Answer from the drawing. Dimensions are ordinates in mm from the lowest x, y and z of the part. Round coordinates to 2 decimals unless told otherwise and drop trailing zeros. Order: outer loops, then holes, each group sorted by start corner. A loop starts at its lowest first (then second) coordinate and runs counter-clockwise, first axis right, second up. Notation, with made-up numbers: (-17.75, -29) -> (5.25, -29) arc R10 cw to (5.25, -18) -> close; hole circle Ø3 at (9, -9). An arc over 180 degrees is marked (long way). Use a Markdown table: item, result. Add a question column.
Item 1: A cutting plane is placed at C-C, the plane y = 100. Determine the outline of the cut face in (x, z).
Item 2: A cutting plane is placed at A-A, the plane y = 40. Determine the outline of the cut face in (x, z).
Item 3: A cutting plane is placed at B-B, the plane x = 48. Determine the outline of the cut face in (y, z).
Item 4: Flat-ended cylindrical pins translate along their axes: P1, Ø5, axis at x = 38.94, y = 66.19, coming from the +Z side; P2, Ø1.6, axis at x = 82, z = 4, coming from the -Y side; P3, Ø3.5, axis at x = 13, z = 4, coming from the +Y side. Find the tip coordinate at first contact, or state that the pin passes through.
Item 5: A cutting plane is placed at D-D, the plane z = 5.5. Give the number of separate pieces and of enclosed holes in the cut face, plus the area to 3 significant figures.
Item 6: Find the intervals of material crossed by L1, parallel to Z at x = 83, y = 16; L2, parallel to Y at x = 48, z = 6.75; L3, parallel to X at y = 76, z = 6.75 (1 decimal), in increasing order. Write a range as [from, to].
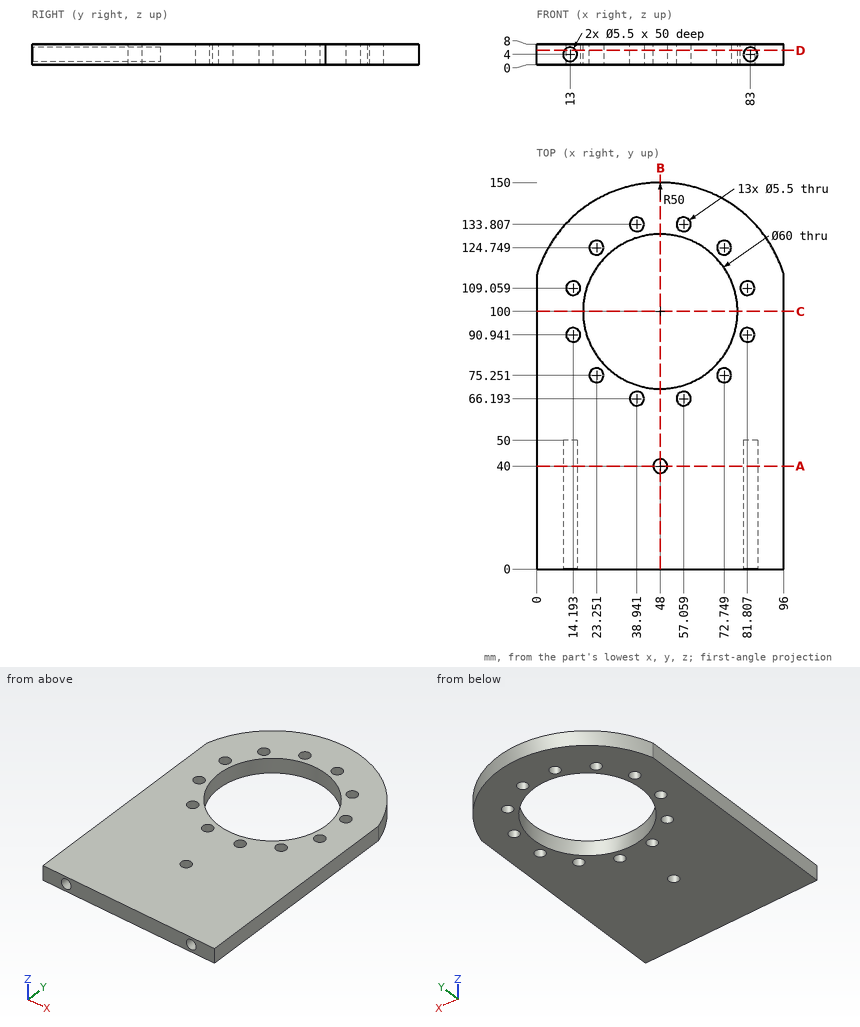
Reported:
| question | item | result |
|---|---|---|
| 1 | outline | (0, 0) -> (18, 0) -> (18, 8) -> (0, 8) -> close; (78, 0) -> (96, 0) -> (96, 8) -> (78, 8) -> close |
| 2 | outline | (0, 0) -> (45.25, 0) -> (45.25, 8) -> (0, 8) -> close; (50.75, 0) -> (96, 0) -> (96, 8) -> (50.75, 8) -> close; hole circle Ø5.5 at (13, 4); hole circle Ø5.5 at (83, 4) |
| 3 | outline | (0, 0) -> (37.25, 0) -> (37.25, 8) -> (0, 8) -> close; (42.75, 0) -> (70, 0) -> (70, 8) -> (42.75, 8) -> close; (130, 0) -> (150, 0) -> (150, 8) -> (130, 8) -> close |
| 4 | P1 | through |
| 4 | P2 | y = 50 |
| 4 | P3 | y = 137.34 |
| 5 | separate pieces | 1 |
| 5 | enclosed holes | 14 |
| 5 | area | 9,890 mm² |
| 6 | L1 | [0, 1.25], [6.75, 8] |
| 6 | L2 | [0, 37.25], [42.75, 70], [130, 150] |
| 6 | L3 | [0, 20.6], [25.9, 30], [66, 70.1], [75.4, 96] |
